Source: CAD feature listing. Evaluate the final solid. Frame: model axes, mm. A direction names the side the tool comes from. Round coordinates to 2 decimals unless told otherwise and drop trailing zeros. Order: outer loops, then holes, each group sorted by start corner. A loop starts at its lowest first (then second) coordinate and runs counter-clockwise, first axis right, second up. Notation, with made-up numbers: M 57,77.5 L 115,77.5 A35 ccw 115,116.5 Z; hole C 49.25,49.5 d7. An arc over 180 degrees is marked long. Answer in a Markdown table with one row per item. Add a question column.
Autodesk Inventor part; units mm, degrees
ref_plane "Work Plane1" through (0, 12.954, 0) normal (0, 1, 0) x (1, 0, 0)
ref_plane "Work Plane2" through (-7.9375, 22.098, -4.7625) normal (0, 1, 0) x (1, 0, 0)
ref_plane "Work Plane3" through (-7.9375, 30.734, -4.7625) normal (0, 1, 0) x (1, 0, 0)
sketch "Sketch1" plane through (0, 0, 0) normal (0, 1, 0) x (-1, 0, 0)
  line L0 (0, 0) -> (16.3071, 0)
  line L1 (16.3071, 0) -> (8.1536, -14.1224)
  line L2 (8.1536, -14.1224) -> (0, 0)
  point P0 (8.1536, 0)
  dimension "d1" = 14.1224
  dimension "d3" = 0
extrude "Extrusion1" add sketch "Sketch1" along normal blind 8.128
sketch "Sketch2" plane through (0, 8.128, 0) normal (0, 1, 0) x (1, 0, 0)
  ellipse E0 centre (-7.9375, 4.7625) end of major axis (-5.2705, 4.7625) minor radius 3.175
  line L0 (-16.3071, 0) -> (0, 0)
  line L1 (0, 0) -> (-8.1536, 14.1224)
  line L2 (-8.1536, 14.1224) -> (-16.3071, 0)
  line L3 (-8.1536, 14.1224) -> (-16.3071, 0)
  dimension "d8" = 2.667
  dimension "d9" = 3.175
ref_plane "Work Plane1" through (0, 12.954, 0) normal (0, 1, 0) x (1, 0, 0)
sketch "Sketch3" plane through (0, 12.954, 0) normal (0, 1, 0) x (1, 0, 0)
  ellipse E0 centre (-7.9375, 4.7625) end of major axis (-7.9375, 8.3185) minor radius 2.794
  point P0 (0, 0)
  dimension "d11" = 2.794
  dimension "d12" = 3.556
  dimension "d13" = 0
  dimension "d14" = 0
loft "Loft1" add profiles "Sketch3", "Sketch2" contours all / E0
ref_plane "Work Plane2" through (-7.9375, 22.098, -4.7625) normal (0, 1, 0) x (1, 0, 0)
sketch "Sketch4" plane through (-7.9375, 22.098, -4.7625) normal (0, 1, 0) x (1, 0, 0)
  ellipse E0 centre (0, 0) end of major axis (0, 4.953) minor radius 3.937
  point P0 (7.9375, -4.7625)
  dimension "d20" = 3.937
  dimension "d21" = 4.953
sketch "Sketch5" plane through (-7.9375, 12.954, -4.7625) normal (0, 1, 0) x (1, 0, 0)
  ellipse E0 centre (0, 0) end of major axis (0, -7.62) minor radius 5.08
  point P0 (7.9375, -4.7625)
  dimension "d22" = 5.08
  dimension "d23" = 7.62
loft "Loft2" add profiles "Sketch5", "Sketch4"
ref_plane "Work Plane3" through (-7.9375, 30.734, -4.7625) normal (0, 1, 0) x (1, 0, 0)
sketch "Sketch7" plane through (-7.9375, 30.734, -4.7625) normal (0, 1, 0) x (1, 0, 0)
  ellipse E0 centre (0, 0) end of major axis (0, 9.652) minor radius 6.858
  point P0 (7.9375, -4.7625)
  dimension "d29" = 6.858
  dimension "d30" = 9.652
loft "Loft3" add profiles "Sketch7" section 1 edges at (-4.0005, 22.098, -4.7625) (-11.8745, 22.098, -4.7625)
sketch "Sketch8" plane through (-7.9375, 30.734, -4.7625) normal (0, 1, 0) x (1, 0, 0)
  ellipse E0 centre (0, 0) end of major axis (0, -9.652) minor radius 6.858
  line L0 (0, 9.652) -> (0, -9.652)
  point P0 (7.9375, -4.7625)
ref_plane "Work Plane4" through (-7.9375, 30.734, -14.4145) normal (-1, 0, 0) x (0, 0, 1)
sketch "Sketch9" plane through (-7.9375, 30.734, -14.4145) normal (-1, 0, 0) x (0, 0, 1)
  line L0 (0, 0) -> (19.304, 0)
  line L1 (9.652, 0) -> (9.652, 7.4025)
  line L2 (6.35, 6.35) -> (6.35, 3.0298)
  arc A0 (9.652, 7.4025) -> (6.35, 6.35) centre (9.1003, 3.4274) ccw
  arc A1 (6.35, 3.0298) -> (9.652, 0) centre (9.391, 3.0298) ccw
  point P0 (14.4145, -30.734)
revolve "Revolution1" add sketch "Sketch9" angle 360 about axis through (-7.9375, 30.734, -4.7625) along (0, 1, 0)
properties part number "femsle" material "PMMA Plastic"
(1) Cut plane A-A (y = 4.5). Return loops of the section in (x, z), and give its area (3 significant figures).
(2) Access query for faces 1 (the face through (-12.29, 4.01, -6.96)), 2 (the face through (-10, 8.128, -2)), 3 (the face through (-4.134, 4.007, -7.16)), 4 (the face through (-8, 4, 0)). Directions: +Z, -Z, +X, -X, +Y, -Y. A direction counts if a zero-diameter tool reaches every point of the face in a straight line with its end or side. Return the directions, or none.
(3) Cut plane B-B (z = -10.75). Count the separate pieces of the cut face and the enclosed holes in it, and give its area (3 significant figures).
(4) Pin query (flat end, axial travel): pin 1 (5 mm diameter, centred on x = -2, y = 5, fed in from -Z); pin 2 (6 mm diameter, centred on x = -5, z = -2, fed in from +Y); pin 3 (4 mm diameter, centred on x = -5, z = -9, fed in from +Y). Return the tip coordinate at first contact, or that it passes through.
(5) Line query: line 1 (Y direction, x = -4.25, z = -6.25); line 2 (Z direction, x = -10.75, y = 7); line 3 (Z direction, x = -7.75, y = 3). Output: solid intervals per line, ascending. Write a range as from..to.
(6) Draft query along Y for faces 5 (the face through (-6.5, 30.734, -4.6)), 6 (the face through (-6.946, 35.401, -7.912)), 7 (the face through (-8, 0, -5)). Return one class per face: +Y half, -Y half, draft (parallel to the pull), parting line (faces both ways), or undercut.
Answer list:
| question | item | result |
|---|---|---|
| 1 | outline | M -16.31,0 L -8.15,-14.12 L 0,0 Z |
| 1 | area | 115 mm² |
| 2 | face 1 | -Z, -X, -Y |
| 2 | face 2 | none |
| 2 | face 3 | -Z, +X, -Y |
| 2 | face 4 | +Z, +X, -X, -Y |
| 3 | separate pieces | 3 |
| 3 | enclosed holes | 0 |
| 3 | area | 102 mm² |
| 4 | pin 1 | z = -7.79 |
| 4 | pin 2 | y = 38.15 |
| 4 | pin 3 | y = 37.21 |
| 5 | line 1 | 0..8.13, 12.95..30.73 |
| 5 | line 2 | -9.63..0 |
| 5 | line 3 | -13.42..0 |
| 6 | face 5 | undercut |
| 6 | face 6 | draft |
| 6 | face 7 | -Y half |
